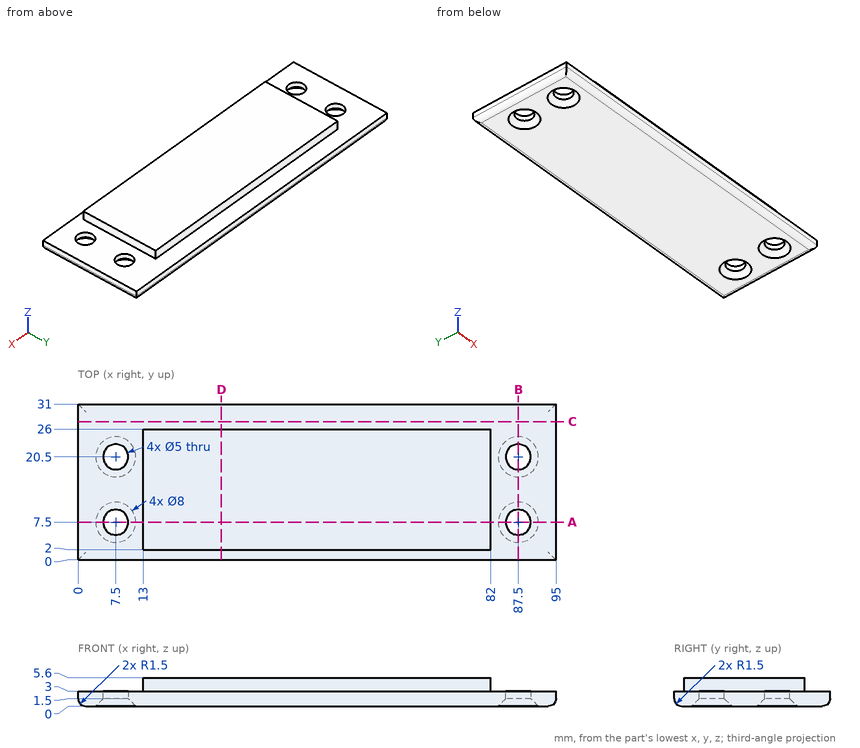
Verification items for this drawing (mm, ordinates from the low corner). Coordinates: 2 decimals unless noted, no trailing zeros. Order: outer loops, then holes, each group sorted by start corner. A loop starts at its lowest first (then second) coordinate and runs counter-clockwise, first axis right, second up. Notation, with made-up numbers: M -13.5,-19 L 33.5,-19 A31 ccw 33.5,20 Z; hole C 28,75.5 d4. An arc over 180 degrees is marked long. Use CSV: the item, a comma, the result in double quotes.
Item 1: Cross-section at A-A on y = 7.5. Record the cut outline in (x, z).
Returned:
outline,"M 0,1.5 A1.5 ccw 1.5,0 L 3.5,0 L 5,1.5 L 5,3 L 0,3 Z; M 10,1.5 L 11.5,0 L 83.5,0 L 85,1.5 L 85,3 L 82,3 L 82,5.6 L 13,5.6 L 13,3 L 10,3 Z; M 90,1.5 L 91.5,0 L 93.5,0 A1.5 ccw 95,1.5 L 95,3 L 90,3 Z"
Item 2: Cross-section at C-C on y = 27.5. Record the cut outline in (x, z).
Returned:
outline,"M 0,1.5 A1.5 ccw 1.5,0 L 93.5,0 A1.5 ccw 95,1.5 L 95,3 L 0,3 Z"
Item 3: Thickness scan on line 1 along Y through (x, z) = (87.5, 2.6); line 2 along Z through (x, y) = (12, 26); line 3 along X through (y, z) = (3.5, 4.15). Record the ranges inside material, lowest first.
Returned:
line 1,"y = 0 to 5, 10 to 18, 23 to 31"
line 2,"z = 0 to 3"
line 3,"x = 13 to 82"
Item 4: Cross-section at B-B on x = 87.5. Record the cut outline in (y, z), then the cut area to 3 significant figures.
Returned:
outline,"M 0,1.5 A1.5 ccw 1.5,0 L 3.5,0 L 5,1.5 L 5,3 L 0,3 Z; M 10,1.5 L 11.5,0 L 16.5,0 L 18,1.5 L 18,3 L 10,3 Z; M 23,1.5 L 24.5,0 L 29.5,0 A1.5 ccw 31,1.5 L 31,3 L 23,3 Z"
area,"57.5 mm2"
Item 5: Cross-section at D-D on x = 28.5. Record the cut outline in (y, z), then the cut area to 3 significant figures.
Returned:
outline,"M 0,1.5 A1.5 ccw 1.5,0 L 29.5,0 A1.5 ccw 31,1.5 L 31,3 L 26,3 L 26,5.6 L 2,5.6 L 2,3 L 0,3 Z"
area,"154 mm2"
Item 6: Gauge pin test, flat ends, axial feed: pin 1 Ø1.3 at (y, z) = (15.5, 4.5) entering from +X; pin 2 Ø0.8 at (y, z) = (8.5, 4.5) entering from -X; pin 3 Ø6.5 at (x, y) = (7.5, 7.5) entering from +Z; pin 4 Ø3 at (x, z) = (33.5, 4) entering from +Y. Record the tip position at first contact, or that the pin passes through.
Returned:
pin 1,"stops at x = 82"
pin 2,"stops at x = 13"
pin 3,"stops at z = 3"
pin 4,"stops at y = 31"
